Source: CAD feature listing. Evaluate the final solid. Frame: model axes, mm. Face numbers are marked on the shaded views. A direction names the side the tool comes from. Give positions to 0.01 mm unless a question says otherwise; leave off trailing zeros. Order: outer loops, then holes, each group sorted by start corner. A loop starts at its lowest first (then second) coordinate and runs counter-clockwise, first axis right, second up.
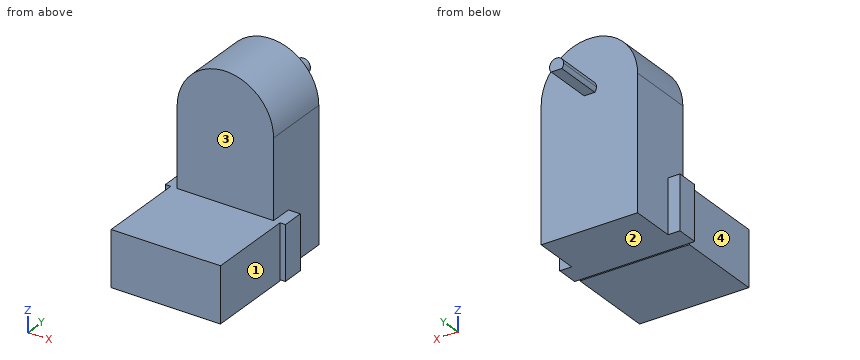
```python
from build123d import *

# Parameters (mm, degrees)
F0_W     = 19.9
F0_H     = 27.35
F1_DEPTH = 13.75
F2_W     = 19.9
F2_H     = 11.15
F3_DEPTH = 18.1
F4_W     = 24.8
F4_H     = 11.15
F5_DEPTH = 4.5
F7_DEPTH = 10


with BuildPart() as f1:
    # F0 (on Front) → F1 (new body)
    with BuildSketch(Plane.XZ):
        with BuildLine():
            ThreePointArc((9.95, 0), (0, 9.95), (-9.95, 0))
            Line((-9.95, 0), (9.95, 0))
        make_face()
        with Locations((0, -13.675)):
            Rectangle(F0_W, F0_H)
    extrude(amount=F1_DEPTH)

    # F2 (on face) → F3 (join)
    with BuildSketch(Plane.XZ.offset(13.75)):
        Polygon((-11.275, -16.2), (-11.275, -27.6), (11.275, -27.6), (11.275, -16.2), (9.95, -16.2), (9.95, -27.35), (-9.95, -27.35), (-9.95, -16.2), align=None)
        with Locations((0, -21.775)):
            Rectangle(F2_W, F2_H)
    extrude(amount=F3_DEPTH)

    # F4 (on face) → F5 (join)
    with BuildSketch(Plane.XZ.offset(13.75)):
        with Locations((0, -21.775)):
            Rectangle(F4_W, F4_H)
    extrude(amount=-F5_DEPTH)

    # F6 (on face) → F7 (join)
    with BuildSketch(Plane(origin=(0, 0, 0), x_dir=(-1, 0, 0), z_dir=(0, 1, 0))):
        with BuildLine():
            ThreePointArc((1.095445, -0.95), (1.358473, -0.507003), (1.45, 0))
            ThreePointArc((1.45, 0), (-0.507003, 1.358473), (-1.095445, -0.95))
            Line((-1.095445, -0.95), (1.095445, -0.95))
        make_face()
    extrude(amount=F7_DEPTH)


solid = f1.part
```
1) Section query A-A, the plane y = -11.5. Return the cut outline in (x, z).
Report:
outline: (-12.4, -27.35) - (12.4, -27.35) - (12.4, -16.2) - (9.95, -16.2) - (9.95, 0) arc R9.95 ccw to (-9.95, 0) - (-9.95, -16.2) - (-12.4, -16.2) - close
2) Section query D-D, the plane x = 0. Return the cut outline in (y, z), and give its area (3 significant figures).
Report:
outline: (-31.85, -27.6) - (-13.75, -27.6) - (-13.75, -27.35) - (0, -27.35) - (0, -0.95) - (10, -0.95) - (10, 1.45) - (0, 1.45) - (0, 9.95) - (-13.75, 9.95) - (-13.75, -16.2) - (-31.85, -16.2) - close
area: 743 mm2
3) Pin query (flat end, axial travel): pin 1 (7 mm diameter, centred on y = -4.5, z = -14.5, fed in from -X); pin 2 (1.1 mm diameter, centred on x = -0.5, y = 2.5, fed in from -Z); pin 3 (15 mm diameter, centred on y = -8, z = -17, fed in from +X); pin 4 (0.9 mm diameter, centred on x = 12, z = -21, fed in from -Y). Return the tip coordinate at first contact, or that it passes through.
Report:
pin 1: stops at x = -9.95
pin 2: stops at z = -0.95
pin 3: stops at x = 12.4
pin 4: stops at y = -13.75
4) Section query C-C, the plane x = 9.25. Return the cut outline in (y, z).
Report:
outline: (-31.85, -27.6) - (-13.75, -27.6) - (-13.75, -27.35) - (0, -27.35) - (0, 3.67) - (-13.75, 3.67) - (-13.75, -16.2) - (-31.85, -16.2) - close
5) Reachability of the marked faces 1, 2, 3 and 4 from +Z, -Z, +X, -X, +Y, -Y: full face, straight path, thin tool, end or side. Return the list, or none.
Report:
face 1: +Z, -Z, +X, -Y
face 2: -Z, +X, -X, +Y
face 3: +Z, +X, -X, -Y
face 4: +Z, -Z, -X, -Y
6) Section query B-B, the plane z = -19. Return the cut outline in (x, y) (3 decimals).
Report:
outline: (-12.4, -13.75) - (-11.275, -13.75) - (-11.275, -31.85) - (11.275, -31.85) - (11.275, -13.75) - (12.4, -13.75) - (12.4, -9.25) - (9.95, -9.25) - (9.95, 0) - (-9.95, 0) - (-9.95, -9.25) - (-12.4, -9.25) - close
7) Material intervals for L1, parallel to Y at x = -3, z = 6.5; L2, parallel to Z at x = 2, y = -27; L3, parallel to Z at x = -10.75, y = -11, sorted ascending.
Report:
L1: y = -13.75 to 0
L2: z = -27.6 to -16.2
L3: z = -27.35 to -16.2
